Geometry: final body of the model. Coordinates: model frame, mm. Give positions to 0.01 mm unless a question says otherwise; leave off trailing zeros. Write each loop counter-clockwise with the first axis right and the second up, starting at its lowest first coordinate (ties: lowest second). Pieces come first, ordered by that corner, then holes. Notation, with made-up numbers: M 4,40 L 30,40 A31 cw 30,78 Z; hole C 25.25,26.25 d8. An arc over 180 degrees is marked long. Use a Markdown table: item, result. Add a question column.
1) Section B-B on x = 852. Return the cut outline in (y, z).
2) Draft query along Y for faces 1 (the flat face through (269.504, 223.14, -650.095)), 2 (the cylindrical face through (895.823, -5.124, -1148.944)), 3 (the cylindrical face through (897.78, -4.68, -1128.95)). Return one class per face: +Y half, -Y half, draft (parallel to the pull), parting line (faces both ways), or undercut.
3) Line query: line 1 (Y direction, x = 796, z = -1055.5); line 2 (Y direction, x = 591, z = -949.5); line 3 (Z direction, x = 186.5, y = 13.5). Output: solid intervals per line, ascending.
4) Section C-C on y = 0. Return the cut outline in (x, z).
5) Pin query (flat end, axial travel): pin 1 (10 mm diameter, centred on y = 76, z = -964.5, fed in from -X); pin 2 (12 mm diameter, centred on x = 59.5, y = 85, fed in from +Z); pin 3 (10 mm diameter, centred on x = 247, y = -89.5, fed in from -Z). Return the tip coordinate at first contact, or that it passes through.
6) Section A-A on y = -130. Return the cut outline in (x, z).
```python
from build123d import *


with BuildPart() as f3:
    # F3: sweep along a path in F0
    with BuildLine(Plane.XZ) as f3_path:
        Line((0, -183.805903785), (139.1482145694, -519.7394105784))
        Line((139.1482145694, -519.7394105784), (396.2605894216, -776.8517854306))
        Line((396.2605894216, -776.8517854306), (732.194096215, -916))
        Line((732.194096215, -916), (1100, -916))
    # F2 (on line) → F3 (sweep)
    with BuildSketch(Plane.YZ.offset(1100)):
        with BuildLine():
            ThreePointArc((213, -916), (0, -1129), (-213, -916))
            Line((-213, -916), (-233, -916))
            ThreePointArc((-233, -916), (0, -1149), (233, -916))
            Line((233, -916), (213, -916))
        make_face()
    sweep(path=f3_path.line, transition=Transition.RIGHT)


solid = f3.part
```
Found:
| question | item | result |
|---|---|---|
| 1 | outline | M -233,-916 A233 ccw 233,-916 L 213,-916 A213 cw -213,-916 Z |
| 2 | face 1 | draft |
| 2 | face 2 | parting line |
| 2 | face 3 | undercut |
| 3 | line 1 | -186.62 to -160.96, 160.96 to 186.62 |
| 3 | line 2 | -216.95 to -195.31, 195.31 to 216.95 |
| 3 | line 3 | -896.05 to -867.71 |
| 4 | outline | M -215.26,-272.97 L -58.38,-651.72 L 264.28,-974.38 L 685.85,-1149 L 1100,-1149 L 1100,-1129 L 689.83,-1129 L 275.61,-957.42 L -41.42,-640.39 L -196.79,-265.32 Z |
| 5 | pin 1 | x = 266.87 |
| 5 | pin 2 | z = -709.2 |
| 5 | pin 3 | z = -937.6 |
| 6 | outline | M -178.64,-257.8 L -24.78,-629.27 L 286.73,-940.78 L 693.73,-1109.36 L 1100,-1109.36 L 1100,-1084.73 L 698.63,-1084.73 L 300.68,-919.89 L -3.89,-615.32 L -155.88,-248.38 Z |
